Can you work these out from the model? Positions are in its coordinate system, mm. A direction names the side the tool comes from. Give positions to 0.01 mm unless a question says otherwise; leave off trailing zeros. Loops run counter-clockwise (first coordinate to the right, second up) from the corner with the lowest first, then second, coordinate; pieces in that order, holes last. Notation, with made-up numbers: (29, -30) -> (79, -30) arc R32 cw to (79, 4) -> close; hole circle Ø7 at (-4.75, 29.5). An arc over 180 degrees is marked (long way). One line per question, with ' | ' between items.
Solid Edge part; units mm, degrees
sketch "Sketch1" plane through (0, 0, 0) normal (0, -1, 0) x (1, 0, 0)
  line L0 (79.375, -3.9161) -> (3.175, 63.5)
  line L1 (3.175, 50.8) -> (3.175, 63.5)
  line L2 (0, 50.8) -> (3.175, 50.8)
  line L3 (0, 0) -> (0, 50.8)
  line L4 (3.175, 0) -> (0, 0)
  line L5 (3.175, 0) -> (79.375, -31.75)
  line L6 (79.375, -31.75) -> (79.375, -3.9161)
extrude "Protrusion1" add sketch "Sketch1" along normal mid plane 3.175
chamfer "Chamfer_1" distance 1.5875 angle 45 2 edges at (41.275, -1.5875, 29.792) (41.275, 1.5875, 29.792)
Q1. If we section it at A-A (y = -1): Write out the boundary of the cut face in (x, z) (3 decimals).
Entries:
outline: (0, 0) -> (3.175, 0) -> (79.375, -31.75) -> (79.375, -5.251) -> (3.175, 62.165) -> (3.175, 50.8) -> (0, 50.8) -> close
Q2. If I drill on probe 1 along Y at (x, z) = (49, 21.5); probe 2 along X at (y, z) = (-0.25, -12) (3 decimals); probe 3 along X at (y, z) = (-0.95, 45), over which ranges is the centre line in solid material (lowest first)? Write a range as from..to.
Entries:
probe 1: -1.09..1.09 | probe 2: 31.975..79.375 | probe 3: 0..22.65
Q3. For pin 1 Ø1 at (x, z) = (44, 27.5) entering from +Y; pin 2 Ø1.5 at (x, y) = (62, -0.5) entering from -Z; pin 3 Ø1 at (x, y) = (2, 0.5) entering from +Z, each with a flat end and sliding along its axis, tell me the tip position at first contact or that it passes through.
Entries:
pin 1: y = 0.41 | pin 2: z = -24.82 | pin 3: z = 50.8
Q4. If we section it at D-D (z = -19.5): Write out the boundary of the cut face in (x, y) (1 decimal), plus the area to 3 significant figures.
Entries:
outline: (50, -1.6) -> (79.4, -1.6) -> (79.4, 1.6) -> (50, 1.6) -> close | area: 93.3 mm²
Q5. On a 3-axis mill with a long thin cutter (end or side, diameter ignored), from which of +Z, -Z, +X, -X, +Y, -Y can I reach the whole of each face in a straight line? I mean faces 1 (the face through (0, 0, 25)), 2 (the face through (2, 0, 0)), 3 (the face through (2, 0, 50.8)). Say none if no direction works.
Entries:
face 1: +Z, -Z, -X, +Y, -Y | face 2: -Z, -X, +Y, -Y | face 3: +Z, -X, +Y, -Y
